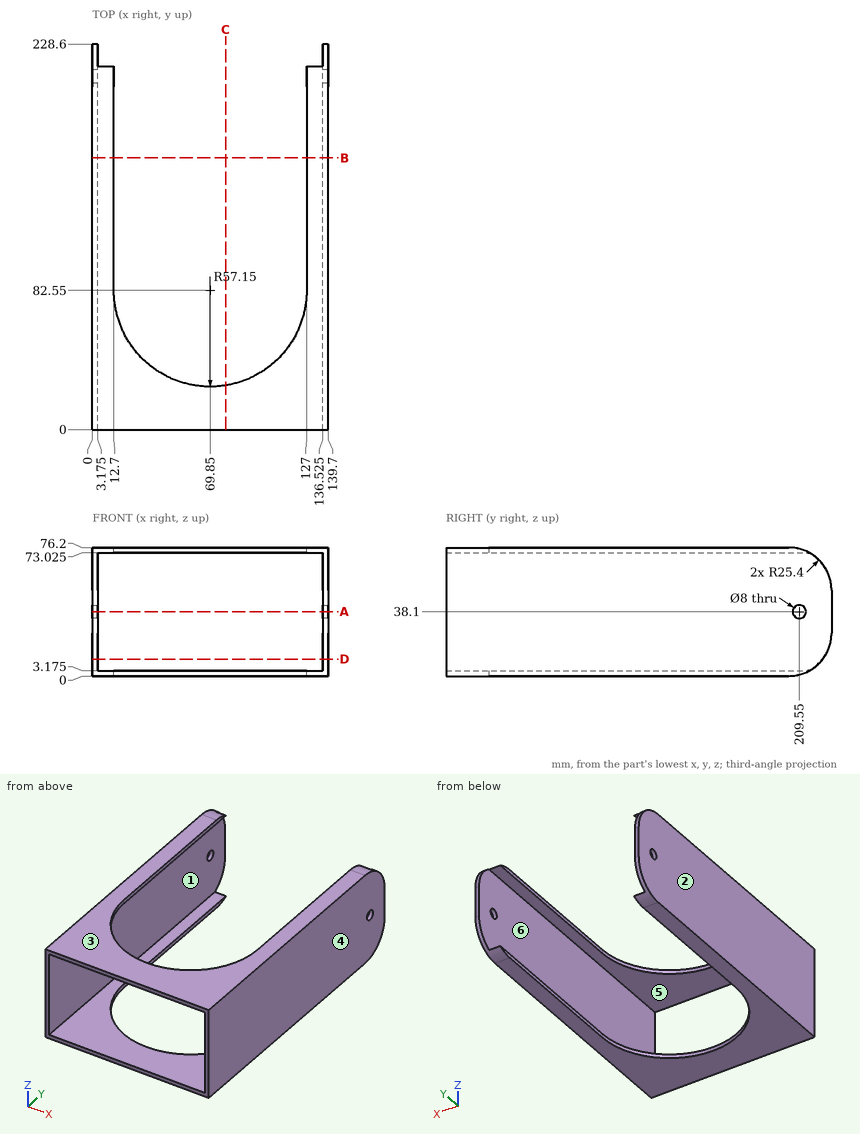
Verification items for this drawing (mm, ordinates from the low corner). A direction names the side the tool comes from. Give positions to 0.01 mm unless a question says otherwise; leave off trailing zeros. Write each loop counter-clockwise with the first axis right and the second up, starting at its lowest first coordinate (ties: lowest second). Pieces come first, ordered by that corner, then holes. Notation, with made-up numbers: (85.25, -25) -> (141.25, -25) arc R17 ccw to (141.25, -14) -> close; hole circle Ø9 at (-20, 10.25). An arc over 180 degrees is marked (long way). Write item = value, one per line.
Item 1: Sectioned sample at A-A on z = 38.1. Record the boundary of the cut face in (x, y) (3 decimals), and give its area (3 significant figures).
Output:
outline = (0, 0) -> (3.175, 0) -> (3.175, 205.55) -> (0, 205.55) -> close; (0, 213.55) -> (3.175, 213.55) -> (3.175, 228.6) -> (0, 228.6) -> close; (136.525, 0) -> (139.7, 0) -> (139.7, 205.55) -> (136.525, 205.55) -> close; (136.525, 213.55) -> (139.7, 213.55) -> (139.7, 228.6) -> (136.525, 228.6) -> close
area = 1,400 mm^2
Item 2: Release check for a two-part mould opening along Z. For the marked faces 3, 4, 5 and 6 record: +Z half, -Z half, draft (parallel to the pull), parting line (faces both ways), or undercut.
Output:
face_3 = +Z half
face_4 = draft
face_5 = undercut
face_6 = undercut
Item 3: Tool access check on the marked faces 1 and 2. Record the directions out of +Z, -Z, +X, -X, +Y, -Y that give a thin tool (end or side, any length) a straight path to the whole face; none if there is none.
Output:
face_1 = +Y, -Y
face_2 = +Z, -Z, -X, +Y, -Y
Item 4: Scan lines: probe 1 along X at (y, z) = (39.5, 11.5) (3 decimals); probe 2 along Y at (x, z) = (0.8, 38.1); probe 3 along Z at (x, y) = (10, 21.5) (3 decimals). Record each from-to range of solid material in increasing order. Write a range as from..to.
Output:
probe_1 = 0..3.175, 136.525..139.7
probe_2 = 0..205.55, 213.55..228.6
probe_3 = 0..3.175, 73.025..76.2
Item 5: Sectioned sample at C-C on x = 79. Record the boundary of the cut face in (y, z) (3 decimals).
Output:
outline = (0, 0) -> (26.137, 0) -> (26.137, 3.175) -> (0, 3.175) -> close; (0, 73.025) -> (26.137, 73.025) -> (26.137, 76.2) -> (0, 76.2) -> close
Item 6: Sectioned sample at B-B on y = 161. Record the boundary of the cut face in (x, z) (3 decimals), and give its area (3 significant figures).
Output:
outline = (0, 0) -> (12.7, 0) -> (12.7, 3.175) -> (3.175, 3.175) -> (3.175, 73.025) -> (12.7, 73.025) -> (12.7, 76.2) -> (0, 76.2) -> close; (127, 0) -> (139.7, 0) -> (139.7, 76.2) -> (127, 76.2) -> (127, 73.025) -> (136.525, 73.025) -> (136.525, 3.175) -> (127, 3.175) -> close
area = 605 mm^2
Item 7: Sectioned sample at D-D on z = 10. Record the boundary of the cut face in (x, y) (3 decimals).
Output:
outline = (0, 0) -> (3.175, 0) -> (3.175, 223.399) -> (0, 223.399) -> close; (136.525, 0) -> (139.7, 0) -> (139.7, 223.399) -> (136.525, 223.399) -> close
